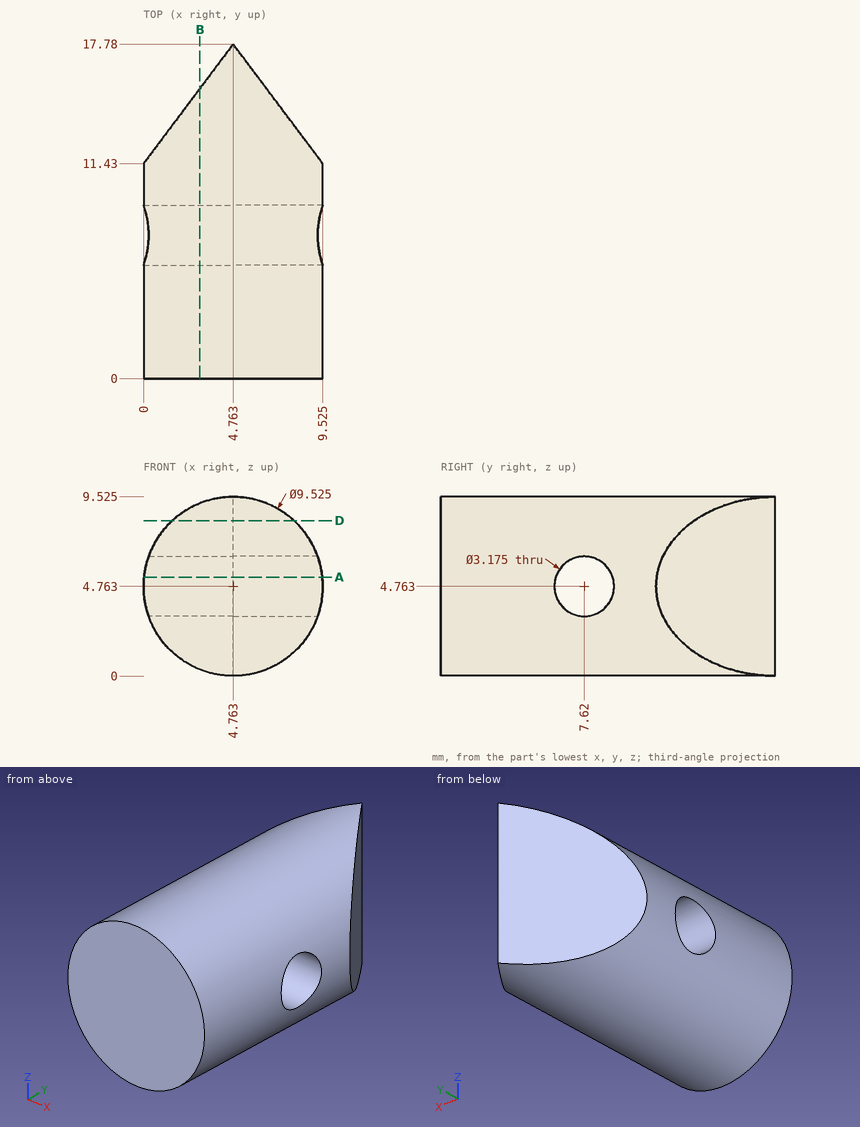
Could you check a few things on this drawing? It's one solid part, dimensions in mm from its lowest x, y, z. Round coordinates to 2 decimals unless told otherwise and drop trailing zeros. Write each loop counter-clockwise with the first axis right and the second up, starting at its lowest first coordinate (ties: lowest second). Pieces come first, ordered by that corner, then holes. Notation, with made-up numbers: (39.25, 45.25) -> (94.25, 45.25) arc R20 cw to (94.25, 83.25) -> close; hole circle Ø3 at (14, -21.75). An arc over 180 degrees is marked (long way). Use a Markdown table: item, result.
1. If we section it at B-B (x = 3): List the corners of the cut face in (y, z) for me (1 decimal).
Answer key:
| item | result |
|---|---|
| outline | (0, 0.3) -> (15.4, 0.3) -> (15.4, 9.2) -> (0, 9.2) -> close; hole circle Ø3.2 at (7.6, 4.8) |
2. Please list where these lines run through material, in increasing order: probe 1 along Y at (x, z) = (8, 6) (1 decimal); probe 2 along Z at (x, y) = (1.25, 8.5) (1 decimal); probe 3 along Y at (x, z) = (1.75, 4.5) (1 decimal).
Answer key:
| item | result |
|---|---|
| probe 1 | y = 0 to 6.6, 8.6 to 13.5 |
| probe 2 | z = 1.5 to 3.4, 6.1 to 8 |
| probe 3 | y = 0 to 6.1, 9.2 to 13.8 |
3. For pin 1 Ø2 at (x, y) = (6.5, 6.5) entering from -Z; pin 2 Ø1 at (x, y) = (4, 6.5) entering from -Z; pin 3 Ø3 at (y, z) = (7.62, 4.76) entering from +X; pin 4 Ø4 at (y, z) = (7.62, 4.76) entering from -X, each with a flat end and sliding along its axis, tell me the tip position at first contact or that it passes through.
Answer key:
| item | result |
|---|---|
| pin 1 | stops at z = 0.06 |
| pin 2 | stops at z = 0.01 |
| pin 3 | passes through |
| pin 4 | stops at x = 0 |
4. If we section it at A-A (z = 5.25): List the corners of the cut face in (x, y) for me (1 decimal).
Answer key:
| item | result |
|---|---|
| outline | (0, 0) -> (9.5, 0) -> (9.5, 6.1) -> (0, 6.1) -> close; (0, 9.1) -> (9.5, 9.1) -> (9.5, 11.5) -> (4.8, 17.8) -> (0, 11.5) -> close |
5. If we section it at D-D (z = 8.25): List the corners of the cut face in (x, y) for me (1 decimal), then the cut area to 3 significant figures.
Answer key:
| item | result |
|---|---|
| outline | (1.5, 0) -> (8, 0) -> (8, 13.5) -> (4.8, 17.8) -> (1.5, 13.5) -> close |
| area | 101 mm^2 |
